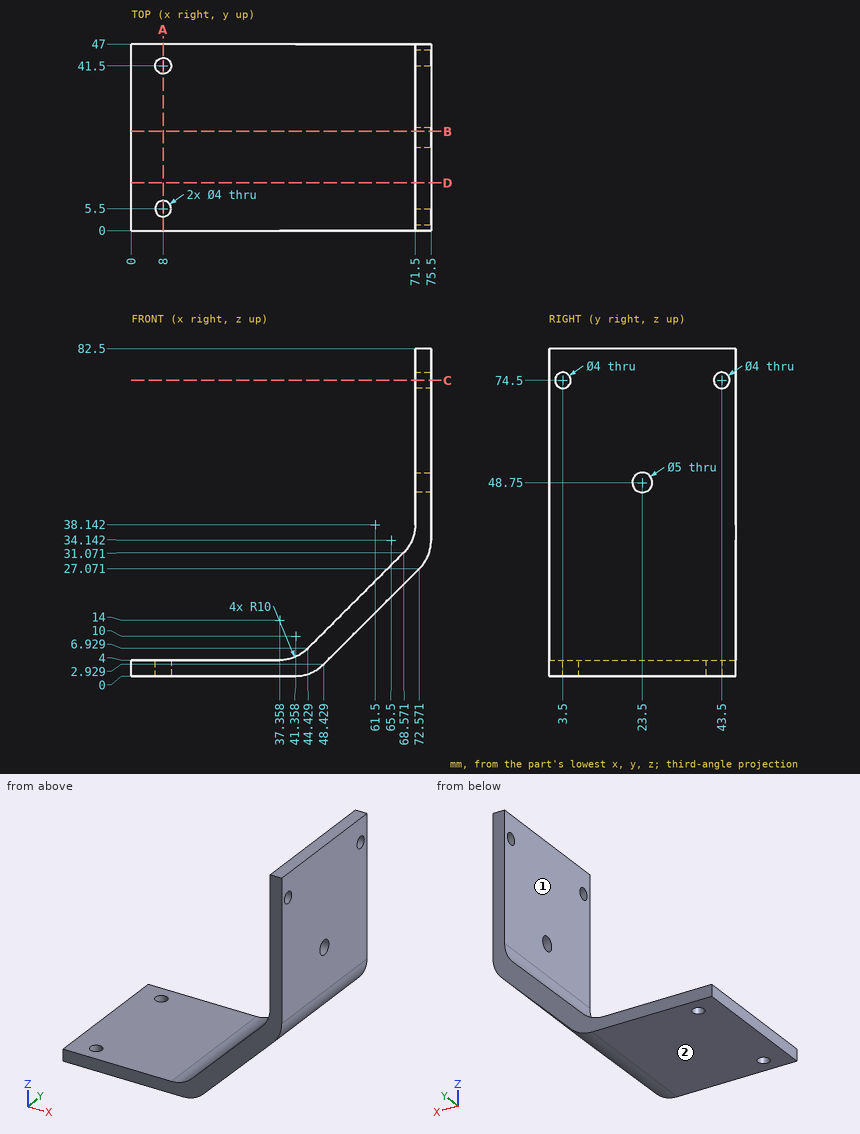
Input: dimensioned drawing with shaded views. Units: mm. Origin: part minimum x, y, z. A direction names the side the tool comes from. Coordinates: 2 decimals unless noted, no trailing zeros. Loops run counter-clockwise (first coordinate to the right, second up) from the corner with the lowest first, then second, coordinate; pieces in that order, holes last.
Q1. Line query: line 1 along Y through (x, z) = (74.25, 74.5); line 2 along Y through (x, z) = (8, 1); line 3 along Y through (x, z) = (74.5, 48.75). Output: solid intervals per line, ascending.
Results are:
line 1: y = 0 to 1.5, 5.5 to 41.5, 45.5 to 47
line 2: y = 0 to 3.5, 7.5 to 39.5, 43.5 to 47
line 3: y = 0 to 21, 26 to 47
Q2. Section B-B, the plane y = 25. Return the cut outline in (x, z), and give its area (3 significant figures).
Results are:
outline: (0, 0) - (41.36, 0) arc R10 ccw to (48.43, 2.93) - (72.57, 27.07) arc R10 ccw to (75.5, 34.14) - (75.5, 46.75) - (71.5, 46.75) - (71.5, 38.14) arc R10 cw to (68.57, 31.07) - (44.43, 6.93) arc R10 cw to (37.36, 4) - (0, 4) - close; (71.5, 50.75) - (75.5, 50.75) - (75.5, 82.5) - (71.5, 82.5) - close
area: 600 mm2
Q3. Section A-A, the plane x = 8. Return the cut outline in (y, z), and give its area (3 significant figures).
Results are:
outline: (0, 0) - (3.5, 0) - (3.5, 4) - (0, 4) - close; (7.5, 0) - (39.5, 0) - (39.5, 4) - (7.5, 4) - close; (43.5, 0) - (47, 0) - (47, 4) - (43.5, 4) - close
area: 156 mm2
Q4. Set-up query: the marked faces 1 and 2. Return all of +Z, -Z, +X, -X, +Y, -Y with unobstructed straight access to the full face (end or side cutting, diameter ignored); none if empty.
Results are:
face 1: +Z, -X, +Y, -Y
face 2: -Z, +X, -X, +Y, -Y
Q5. Contact query for flat-ended pins moving along their axis: pin 1 (5 mm diameter, centred on y = 3.5, z = 74.5, fed in from -X); pin 2 (10 mm diameter, centred on y = 42, z = 32.5, fed in from -X); pin 3 (1.5 mm diameter, centred on x = 48, y = 25, fed in from +Z); pin 4 (2.5 mm diameter, centred on x = 8, y = 41.5, fed in from +Z). Output: stop coordinate, or through.
Results are:
pin 1: stops at x = 71.5
pin 2: stops at x = 65
pin 3: stops at z = 11.25
pin 4: passes through
Q6. Section C-C, the plane z = 74.5. Return the cut outline in (x, y), and give its area (3 significant figures).
Results are:
outline: (71.5, 0) - (75.5, 0) - (75.5, 1.5) - (71.5, 1.5) - close; (71.5, 5.5) - (75.5, 5.5) - (75.5, 41.5) - (71.5, 41.5) - close; (71.5, 45.5) - (75.5, 45.5) - (75.5, 47) - (71.5, 47) - close
area: 156 mm2
Q7. Section D-D, the plane y = 12. Return the cut outline in (x, z).
Results are:
outline: (0, 0) - (41.36, 0) arc R10 ccw to (48.43, 2.93) - (72.57, 27.07) arc R10 ccw to (75.5, 34.14) - (75.5, 82.5) - (71.5, 82.5) - (71.5, 38.14) arc R10 cw to (68.57, 31.07) - (44.43, 6.93) arc R10 cw to (37.36, 4) - (0, 4) - close
